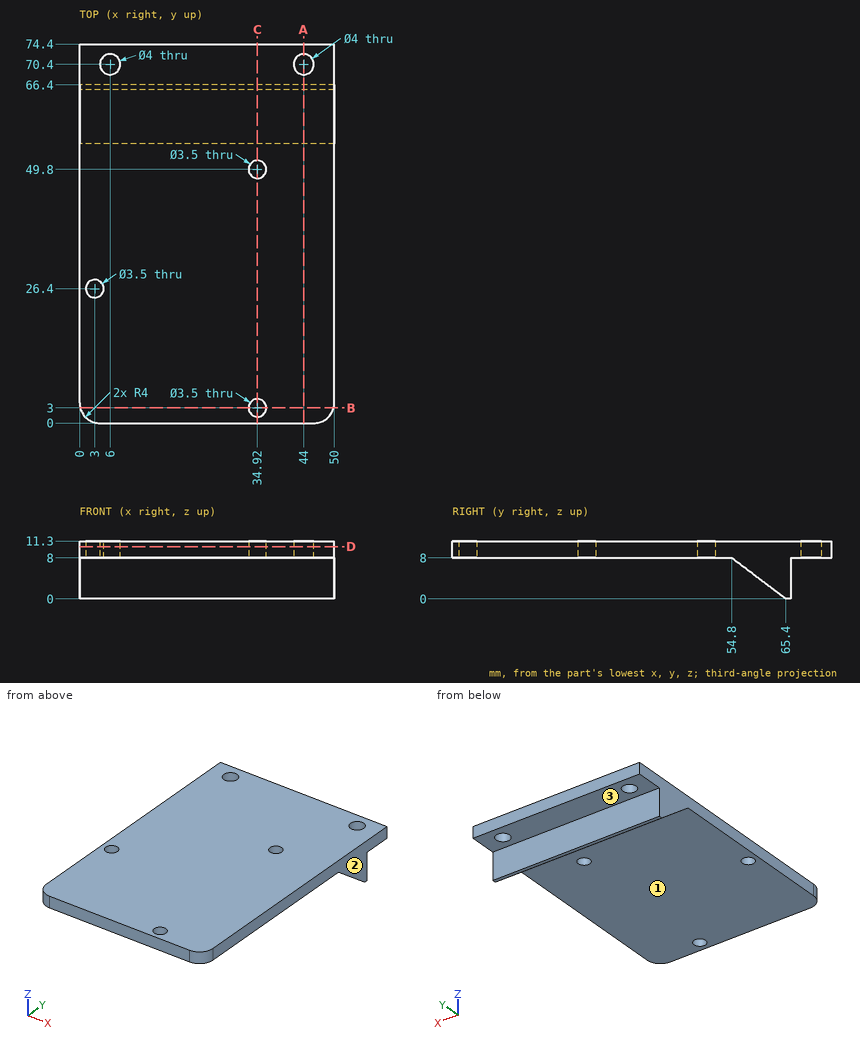
Study the drawing (mm; zero at the part's minimum x, y, z) and answer. A direction names the side the tool comes from. Give positions to 0.01 mm unless a question says otherwise; leave off trailing zeros. Order: outer loops, then holes, each group sorted by start corner. A loop starts at its lowest first (then second) coordinate and runs counter-clockwise, first axis right, second up. Notation, with made-up numbers: (-15.75, 69.25) -> (22.25, 69.25) arc R22 cw to (22.25, 85.25) -> close; hole circle Ø11 at (48.25, -31). An arc over 180 degrees is marked (long way). Write item = value, one per line.
1. Given pin 1 (2 mm diameter, centred on x = 11, y = 51, fed in from -Z); pin 2 (1 mm diameter, centred on x = 37.5, z = 4, fed in from +Y); pin 3 (2 mm diameter, centred on x = 40.5, z = 5.5, fed in from -Y), each flat-ended and moving along its own axis, determine where each tip first touches the part or whether it passes through.
Numbers:
pin_1 = 8
pin_2 = 66.4
pin_3 = 56.79
2. For the marked faces 1, 2 and 3, determine the directions among +Z, -Z, +X, -X, +Y, -Y from which every point of the face is accessible in a straight line to the end or side of a thin tool.
Numbers:
face_1 = -Z, +X, -X, -Y
face_2 = +Z, -Z, +X, +Y, -Y
face_3 = -Z, +X, -X, +Y
3. A cutting plane is placed at A-A, the plane x = 44. Write down the section's boundary in (y, z).
Numbers:
outline = (0, 8) -> (54.8, 8) -> (65.4, 0) -> (66.4, 0) -> (66.4, 8) -> (68.4, 8) -> (68.4, 11.3) -> (0, 11.3) -> close; (72.4, 8) -> (74.4, 8) -> (74.4, 11.3) -> (72.4, 11.3) -> close
4. A cutting plane is placed at B-B, the plane y = 3. Write down the section's boundary in (x, z).
Numbers:
outline = (0.13, 8) -> (33.17, 8) -> (33.17, 11.3) -> (0.13, 11.3) -> close; (36.67, 8) -> (49.87, 8) -> (49.87, 11.3) -> (36.67, 11.3) -> close
5. A cutting plane is placed at D-D, the plane z = 10.25. Write down the section's boundary in (x, y), and give its area (3 significant figures).
Numbers:
outline = (0, 4) arc R4 ccw to (4, 0) -> (46, 0) arc R4 ccw to (50, 4) -> (50, 74.4) -> (0, 74.4) -> close; hole circle Ø3.5 at (3, 26.4); hole circle Ø4 at (6, 70.4); hole circle Ø3.5 at (34.92, 3); hole circle Ø3.5 at (34.92, 49.8); hole circle Ø4 at (44, 70.4)
area = 3,660 mm²
6. A cutting plane is placed at C-C, the plane x = 34.92. Write down the section's boundary in (y, z), and give its area (3 significant figures).
Numbers:
outline = (0, 8) -> (1.25, 8) -> (1.25, 11.3) -> (0, 11.3) -> close; (4.75, 8) -> (48.05, 8) -> (48.05, 11.3) -> (4.75, 11.3) -> close; (51.55, 8) -> (54.8, 8) -> (65.4, 0) -> (66.4, 0) -> (66.4, 8) -> (74.4, 8) -> (74.4, 11.3) -> (51.55, 11.3) -> close
area = 273 mm²
7. Straight lines are drawn through the part: line 1 along Y through (x, z) = (6, 10.45); line 2 along X through (y, z) = (70.4, 10.35); line 3 along Z through (x, y) = (30, 34). For each, find the intervals that lie inside material, in ascending order.
Numbers:
line_1 = 0 to 68.4, 72.4 to 74.4
line_2 = 0 to 4, 8 to 42, 46 to 50
line_3 = 8 to 11.3
